Here's how the part is built. I have some questions about the finished solid (model axes, mm). A direction names the side the tool comes from. Coordinates: 2 decimals unless noted, no trailing zeros. Write each loop counter-clockwise with the first axis right and the second up, starting at its lowest first coordinate (ties: lowest second). Pieces come first, ordered by that corner, then holes.
Item 1: Please list where these lines run through material, in increasing order: line 1 (Y direction, x = -1.5, z = 23); line 2 (Z direction, x = 25.5, y = -7.5); line 3 (Z direction, x = 10, y = 45).
Item 2: I want a section at C-C (z = 24.5). Please give me the cut outline in (x, y).
Item 3: I'm going to push flat-ended pins straight in: P1, Ø5, axis at x = 1, z = 47.5, coming from the -Y side; P2, Ø1, axis at x = 6, y = -40, coming from the +Z side; P3, Ø6, axis at y = -11.5, z = 24.5, coming from the -X side. Where does each tip first touch, or does it pass through?
Item 4: I want a section at A-A (y = 0). Please give me the cut outline in (x, z).
Item 5: For faces 1 (the face through (-25.9, 19.8, -6)), 2 (the face through (13.17, 20.66, 93.63)), 3 (the face through (-10.95, -49.3, 42.15)), which set-ups out of +Z, -Z, +X, -X, +Y, -Y let a thin tool reach every point of the face, with its end or its side?
Item 6: I want a section at D-D (z = 69.5). Please give me the cut outline in (x, y).
from build123d import *

# Parameters (mm, degrees)
F0_R     = 50.5
F1_DEPTH = 85
F2_R     = 17.5
F3_R     = 24.5
F4_DEPTH = 20
F5_R     = 2.5
F6_R     = 32.6
F7_DEPTH = 12.1


with BuildPart() as f1:
    # F0 (on Top) → F1 (new body)
    with BuildSketch(Plane.XY):
        Circle(F0_R)
    extrude(amount=F1_DEPTH)

    # F2
    f2_edges = [f1.edges().sort_by_distance(p)[0] for p in [
        (50.5, 0, 42.5),
        (-50.5, 0, 0),
        (-50.5, 0, 85),
    ]]
    fillet(f2_edges, radius=F2_R)

    # F3 (on face) → F4 (join)
    with BuildSketch(Plane.XY.offset(85)):
        Circle(F3_R)
    extrude(amount=F4_DEPTH)

    # F5
    f5_edges = [f1.edges().sort_by_distance(p)[0] for p in [
        (-24.5, 0, 105),
    ]]
    fillet(f5_edges, radius=F5_R)

    # F6 (on face) → F7 (join)
    with BuildSketch(Plane(origin=(0, 0, 0), x_dir=(1, 0, 0), z_dir=(0, 0, -1))):
        Circle(F6_R)
    extrude(amount=F7_DEPTH)


solid = f1.part
Answer:
1. line 1: y = -50.48 to 50.48
1. line 2: z = -12.1 to 85
1. line 3: z = 5.89 to 79.11
2. outline: circle Ø101 at (0, 0)
3. P1: stops at y = -50.5
3. P2: stops at z = 83.56
3. P3: stops at x = -49.78
4. outline: (-50.5, 17.5) arc R17.5 ccw to (-33, 0) - (-32.6, 0) - (-32.6, -12.1) - (32.6, -12.1) - (32.6, 0) - (33, 0) arc R17.5 ccw to (50.5, 17.5) - (50.5, 67.5) arc R17.5 ccw to (33, 85) - (24.5, 85) - (24.5, 102.5) arc R2.5 ccw to (22, 105) - (-22, 105) arc R2.5 ccw to (-24.5, 102.5) - (-24.5, 85) - (-33, 85) arc R17.5 ccw to (-50.5, 67.5) - close
5. face 1: -Z
5. face 2: +Z
5. face 3: +Z, -Z
6. outline: circle Ø100.77 at (0, 0)
